from build123d import *

# Parameters (mm, degrees)
F0_R       = 32.7181038806
F0_R_2     = 2.3607355304
F1_DEPTH   = 25.4
F2_DEPTH   = 64.008
F3_T       = -2.54
F5_R       = 42.4039305663
F6_DEPTH   = 25.4
F7_DEPTH   = 77.724
F8_R       = 42.4039305663
F7_FACE_R  = 42.4039305663
F6_FACE1_R = 42.4039305663
F9_DEPTH   = 127
F10_R      = 37.8949269506
F11_DEPTH  = 173.228
F12_DEPTH  = 279.908


with BuildPart() as f1:
    # F0 (on Top) → F1 (new body)
    with BuildSketch(Plane.XY):
        Circle(F0_R)
        Circle(F0_R_2, mode=Mode.SUBTRACT)
    extrude(amount=F1_DEPTH)

    # F2 (add): a face of the model
    f2_faces = [f1.faces().sort_by_distance(p)[0] for p in [
        (-31.7926961558, 0, 25.4),
    ]]
    extrude(f2_faces, amount=F2_DEPTH)

    # F3
    f3_openings = [f1.faces().sort_by_distance(p)[0] for p in [
        (-31.792696, 0, 89.408),
    ]]
    offset(amount=F3_T, openings=f3_openings)


with BuildPart() as f6:
    # F5 (on Top) → F6 (new body)
    with BuildSketch(Plane.XY):
        Circle(F5_R)
    extrude(amount=F6_DEPTH)

    # F7 (add): a face of the model
    f7_faces = [f6.faces().sort_by_distance(p)[0] for p in [
        (0, 0, 25.4),
    ]]
    extrude(f7_faces, amount=F7_DEPTH)

    # F8 (on face) + F7_face (on face) + F6_face1 (on face) → F9 (join)
    with BuildSketch(Plane.XY.offset(103.124)):
        Circle(F8_R)
    with BuildSketch(Plane.XY.offset(103.124)):
        Circle(F7_FACE_R)
    with BuildSketch(Plane(origin=(0, 0, 0), x_dir=(1, 0, 0), z_dir=(0, 0, -1))):
        Circle(F6_FACE1_R)
    extrude(amount=F9_DEPTH, dir=(0, 0, 1))

    # F10 (on Top) → F11 (join)
    with BuildSketch(Plane.XY):
        Circle(F10_R)
    extrude(amount=F11_DEPTH)

    # F12 (add): a face of the model
    f12_faces = [f6.faces().sort_by_distance(p)[0] for p in [
        (0, 0, 0),
    ]]
    extrude(f12_faces, amount=-F12_DEPTH)


solid = f6.part
Check sheet for the modelled part. Datum: model origin and axes. Units: mm. Give positions to 0.01 mm unless a question says otherwise; leave off trailing zeros. Order: outer loops, then holes, each group sorted by start corner. A loop starts at its lowest first (then second) coordinate and runs counter-clockwise, first axis right, second up. Notation, with made-up numbers: M 33,70 L 63,70 A25 ccw 63,106 Z; hole C -14,10 d1. An arc over 180 degrees is marked long. Answer as CSV lines item,"result". Start each with the question number.
Item 1: Gauge pin test, flat ends, axial feed: P1, Ø1, axis at y = -5, z = 149.5, coming from the +X side; P2, Ø5, axis at x = -11.5, y = 17.5, coming from the -Z side; P3, Ø6, axis at x = -8, z = 144, coming from the +Y side; P4, Ø10, axis at y = 17, z = 127.5, coming from the -X side. Record the tip position at first contact, or that the pin passes through.
Item 2: Thickness scan on line 1 (X direction, y = -0.5, z = 227.5); line 2 (Y direction, x = -27, z = 78.5); line 3 (Y direction, x = -4, z = 71.5). Record the ranges inside material, lowest first. Write a range as [from, to].
Item 3: Cross-section at A-A on z = 256. Enter the section's corners in (x, y).
Item 4: Cross-section at B-B on x = -29. Enter the section's corners in (y, z).
Item 5: Cross-section at C-C on y = 14. Enter the section's corners in (x, z).
Established:
1,P1,"stops at x = 42.16"
1,P2,"stops at z = 0"
1,P3,"stops at y = 42.11"
1,P4,"stops at x = -40.67"
2,line 1,"x = [-42.4, 42.4]"
2,line 2,"y = [-32.7, 32.7]"
2,line 3,"y = [-42.21, 42.21]"
3,outline,"C 0,0 d84.81"
4,outline,"M -30.94,0 L 30.94,0 L 30.94,279.91 L -30.94,279.91 Z"
5,outline,"M -40.03,0 L 40.03,0 L 40.03,279.91 L -40.03,279.91 Z"
